```python
from build123d import *

# Parameters (mm, degrees)
SKETCH_1_R          = 21
SKETCH_1_R_2        = 16
EXTRUDE_1_DEPTH     = 70
EXTRUDE_START       = 7
SKETCH_3_R          = 21
EXTRUDE_2_DEPTH     = 7
SKETCH_4_R          = 10
EXTRUDE_3_DEPTH     = 109
FILLET_4_R          = 3
SKETCH_5_W          = 7.833460296
SKETCH_5_H          = 29.006841396
CUT_EXTRUDE_1_DEPTH = 38
SKETCH_9_R          = 2.5
CUT_EXTRUDE_3_DEPTH = 77.5
EXTRUDE_START_2     = 25
SKETCH_10_R         = 16
EXTRUDE_4_DEPTH     = 25
FILLET_5_R          = 5
SKETCH_11_R         = 25
SKETCH_11_R_2       = 16
EXTRUDE_5_DEPTH     = 5
SKETCH_14_R         = 15
EXTRUDE_6_DEPTH     = 21
SKETCH_7_R          = 4.000000002
CUT_EXTRUDE_2_DEPTH = 77.5
SKETCH_15_W         = 9.449953832
SKETCH_15_H         = 32.068314676
CUT_EXTRUDE_4_DEPTH = 25.5


with BuildPart() as part:
    # Эскиз1 → Вытянуть1 (new body)
    with BuildSketch(Plane(origin=(0, 0, 0), x_dir=(1, 0, 0), z_dir=(0, 1, 0))):
        with Locations(Location((0, 0, 0), (0, 0, 270))):
            Circle(SKETCH_1_R)
        with Locations(Location((0, 0, 0), (0, 0, 270))):
            Circle(SKETCH_1_R_2, mode=Mode.SUBTRACT)
    extrude(amount=EXTRUDE_1_DEPTH)

    # Эскиз3 → Вытянуть2 (add)
    with BuildSketch(Plane.XZ.offset(EXTRUDE_START)):
        with Locations(Location((0, 0, 0), (0, 0, 270))):
            Circle(SKETCH_3_R)
    extrude(amount=-EXTRUDE_2_DEPTH)

    # Эскиз4 → Вытянуть3 (add)
    with BuildSketch(Plane.XZ.offset(7)):
        with Locations(Location((0, 0, 0), (0, 0, 270))):
            Circle(SKETCH_4_R)
    extrude(amount=EXTRUDE_3_DEPTH)

    # Скругление4
    fillet_4_edges = [part.edges().sort_by_distance(p)[0] for p in [
        (0, -116, 10),
    ]]
    fillet(fillet_4_edges, radius=FILLET_4_R)

    # Эскиз5 → Вырез-Вытянуть1 (cut, symmetric)
    with BuildSketch(Plane.XY):
        with Locations((-12.931100354, -108.165099948)):
            Rectangle(SKETCH_5_W, SKETCH_5_H)
        with Locations((12.931100354, -108.165099948)):
            Rectangle(SKETCH_5_W, SKETCH_5_H)
    extrude(amount=CUT_EXTRUDE_1_DEPTH, both=True, mode=Mode.SUBTRACT)

    # Эскиз9 → Вырез-Вытянуть3 (cut, symmetric)
    with BuildSketch(Plane(origin=(-27.016636389, 0, -1.023584716), x_dir=(-0.03786003720910068, 0, 0.9992830517838905), z_dir=(-0.9992830517838904, 0, -0.03786003720910067))):
        with Locations(Location((-3.61e-07, -109.358787083, 0), (0, 0, 180))):
            Circle(SKETCH_9_R)
    extrude(amount=CUT_EXTRUDE_3_DEPTH, both=True, mode=Mode.SUBTRACT)

    # Эскиз10 → Вытянуть4 (add)
    with BuildSketch(Plane.XZ.offset(7).offset(EXTRUDE_START_2)):
        with Locations(Location((0, 0, 0), (0, 0, 90))):
            Circle(SKETCH_10_R)
    extrude(amount=-EXTRUDE_4_DEPTH)

    # Скругление5
    fillet_5_edges = [part.edges().sort_by_distance(p)[0] for p in [
        (0, -7, -16),
    ]]
    fillet(fillet_5_edges, radius=FILLET_5_R - 0.0001)  # a hair under: the kernel refuses the full size

    # Эскиз11 → Вытянуть5 (add)
    with BuildSketch(Plane(origin=(0, 70, 0), x_dir=(1, 0, 0), z_dir=(0, 1, 0))):
        with Locations(Location((0, 0, 0), (0, 0, 270))):
            Circle(SKETCH_11_R)
        with Locations(Location((0, 0, 0), (0, 0, 90))):
            Circle(SKETCH_11_R_2, mode=Mode.SUBTRACT)
    extrude(amount=EXTRUDE_5_DEPTH)

    # Эскиз14 → Вытянуть6 (add)
    with BuildSketch(Plane.XZ.offset(61)):
        with Locations(Location((0, 0, 0), (0, 0, 90))):
            Circle(SKETCH_14_R)
    extrude(amount=EXTRUDE_6_DEPTH)

    # Эскиз7 → Вырез-Вытянуть2 (cut, symmetric)
    with BuildSketch(Plane(origin=(-26.476014958, 0, -1.003102084), x_dir=(-0.037860037209100694, 0, 0.9992830517838905), z_dir=(-0.9992830517838904, 0, -0.03786003720910069))):
        with Locations((-0.488081216, -71.29866531)):
            Circle(SKETCH_7_R)
    extrude(amount=CUT_EXTRUDE_2_DEPTH, both=True, mode=Mode.SUBTRACT)

    # Эскиз15 → Вырез-Вытянуть4 (cut, symmetric)
    with BuildSketch(Plane.XY):
        with Locations((-18.736164954, -71.146680529)):
            Rectangle(SKETCH_15_W, SKETCH_15_H)
        with Locations((18.736164954, -71.146680529)):
            Rectangle(SKETCH_15_W, SKETCH_15_H)
    extrude(amount=CUT_EXTRUDE_4_DEPTH, both=True, mode=Mode.SUBTRACT)


solid = part.part
```
The model under review builds one solid part; all positions refer to its coordinate system, in mm. A direction names the side the tool comes from. Round coordinates to 2 decimals unless told otherwise and drop trailing zeros. Loops run counter-clockwise (first coordinate to the right, second up) from the corner with the lowest first, then second, coordinate; pieces in that order, holes last. Notation, with made-up numbers: (11.5, 4.25) - (32.5, 4.25) arc R12 ccw to (32.5, 27.25) - close; hole circle Ø11 at (61, -35.75). An arc over 180 degrees is marked (long way). Use a Markdown table: item, result. Add a question column.
Q1. Insertion check: pin 1 Ø12 at (y, z) = (13, 13) entering from +X; pin 2 Ø8.5 at (y, z) = (-74, -1.5) entering from -X; pin 3 Ø3 at (x, z) = (-8, 15) entering from -Y. Each pin has a flat end and moves straight along its axis. Give the tip position at first contact, or say it passes through.
Q2. The part is to be moulded in two halves that separate along Y. For faces 4 (the face through (-0.287, -67.926, 1.653)), 5 (the face through (-10, -61, -4)), 6 (the face through (9.014, -105, 0)), 7 (the face through (0, 0, 0)), say which applies: pulls with the +Y half, pulls with the -Y half, needs draft (parallel to the pull), parting line crosses it, or undercut.
Q3. Add section A-A (y = 59). State the section outline as (x, z) points, plus the area to 3 significant figures.
Q4. Add section B-B (y = -98). State the section outline as (x, z) points.
Q5. Machinability: for faces 1 (the face through (14.011, -74, 4)), 2 (the face through (-9.76, -46.3, 2.17)), 3 (the face through (-9.014, -105, 0)), which of the approach directions +Z, -Z, +X, -X, +Y, -Y give a long, thin tool a straight path to every point of the face, cutting with its end or side? Answer none if there is none.
Q6. Add section C-C (z = 0). State how many separate pieces and enclosed holes the cut face has, plus the area to 3 significant figures.
Q7. For probe 1 along X at (y, z) = (20, 0); probe 2 along Y at (x, z) = (-1.5, 10); probe 3 along Y at (x, z) = (1, 1), list the stretches that pass through material, from the lowest coordinate up.
Worked answers:
| question | item | result |
|---|---|---|
| 1 | pin 1 | x = 19.8 |
| 1 | pin 2 | x = -14.01 |
| 1 | pin 3 | y = -32 |
| 2 | face 4 | undercut |
| 2 | face 5 | undercut |
| 2 | face 6 | needs draft |
| 2 | face 7 | pulls with the +Y half |
| 3 | outline | circle Ø42 at (0, 0); hole circle Ø32 at (0, 0) |
| 3 | area | 581 mm² |
| 4 | outline | (-9.01, -4.33) arc R10 ccw to (9.01, -4.33) - (9.01, 4.33) arc R10 ccw to (-9.01, 4.33) - close |
| 5 | face 1 | +Z, -Z, +X, -Y |
| 5 | face 2 | none |
| 5 | face 3 | +Z, -Z, -X, -Y |
| 6 | separate pieces | 3 |
| 6 | enclosed holes | 0 |
| 6 | area | 3,390 mm² |
| 7 | probe 1 | -21 to -16, 16 to 21 |
| 7 | probe 2 | -82 to -61, -32 to 0 |
| 7 | probe 3 | -116 to -111.67, -107.05 to -75.03, -67.57 to 0 |
